Autodesk Inventor part; units mm, degrees
ref_plane "YZ Plane" through (0, 0, 0) normal (1, 0, 0) x (0, 1, 0)
ref_plane "XZ Plane" through (0, 0, 0) normal (0, 1, 0) x (-1, 0, 0)
ref_plane "XY Plane" through (0, 0, 0) normal (0, 0, 1) x (1, 0, 0)
sketch "Sketch2" plane through (0, 0, 0) normal (0, 1, 0) x (-1, 0, 0)
  line L0 (-75, -30) -> (75, -30)
  line L1 (75, -30) -> (75, 30)
  line L2 (75, 30) -> (-75, 30)
  line L3 (-75, 30) -> (-75, -30)
  line L4 (-75, -30) -> (75, 30) construction
  line L5 (75, -30) -> (-75, 30) construction
  line L6 (-84, -39) -> (84, -39)
  line L7 (84, -39) -> (84, 39)
  line L8 (84, 39) -> (-84, 39)
  line L9 (-84, 39) -> (-84, -39)
  line L10 (-84, -39) -> (84, 39) construction
  line L11 (84, -39) -> (-84, 39) construction
  point P0 (0, 0)
  dimension "d0" = 150
  dimension "d1" = 60
  dimension "d4" = 9
  dimension "d5" = 9
  dimension "d53" = 168
  dimension "d54" = 78
extrude "Extrusion1" add sketch "Sketch2" along normal blind 10
sketch "Sketch4" plane through (0, 10, 0) normal (0, 1, 0) x (1, 0, 0)
  line L0 (-84, 39) -> (-84, -39) construction
  line L1 (-84, -39) -> (84, -39) construction
  line L2 (84, -39) -> (84, 39) construction
  line L3 (84, 39) -> (-84, 39) construction
  line L4 (75, 30) -> (75, -30) construction
  line L5 (75, -30) -> (-75, -30) construction
  line L6 (-75, -30) -> (-75, 30) construction
  line L7 (-75, 30) -> (75, 30) construction
  line L8 (-75, 30) -> (75, 30)
  line L9 (75, 30) -> (75, -30)
  line L10 (75, -30) -> (-75, -30)
  line L11 (-75, -30) -> (-75, 30)
  line L12 (-75, 30) -> (75, -30) construction
  line L13 (75, 30) -> (-75, -30) construction
  line L14 (-79, 34) -> (79, 34)
  line L15 (79, 34) -> (79, -34)
  line L16 (79, -34) -> (-79, -34)
  line L17 (-79, -34) -> (-79, 34)
  line L18 (-79, 34) -> (79, -34) construction
  line L19 (79, 34) -> (-79, -34) construction
  point P0 (0, 0)
  dimension "d8" = 4
  dimension "d9" = 4
extrude "Extrusion2" cut sketch "Sketch4" against normal blind 1
sketch "Sketch7" plane through (0, 9, 0) normal (0, 1, 0) x (1, 0, 0)
  line L0 (79, -34) -> (-79, -34) construction
  line L1 (79, 34) -> (79, -34) construction
  line L2 (-79, 34) -> (79, 34) construction
  line L3 (-79, -34) -> (-79, 34) construction
  line L4 (75, 30) -> (-75, 30) construction
  line L5 (75, -30) -> (75, 30) construction
  line L6 (-75, -30) -> (75, -30) construction
  line L7 (-75, 30) -> (-75, -30) construction
  line L8 (-76, 31) -> (76, 31)
  line L9 (76, 31) -> (76, -31)
  line L10 (76, -31) -> (-76, -31)
  line L11 (-76, -31) -> (-76, 31)
  line L12 (-76, 31) -> (76, -31) construction
  line L13 (76, 31) -> (-76, -31) construction
  line L14 (-79, 34) -> (79, 34)
  line L15 (79, 34) -> (79, -34)
  line L16 (79, -34) -> (-79, -34)
  line L17 (-79, -34) -> (-79, 34)
  line L18 (-79, 34) -> (79, -34) construction
  line L19 (79, 34) -> (-79, -34) construction
  point P0 (0, 0)
  dimension "d15" = 3
  dimension "d16" = 3
extrude "Extrusion3" cut sketch "Sketch7" against normal blind 2.5
fillet "Fillet1" radius 2 8 edges at (76, 7.75, 31) (-76, 7.75, 31) (-76, 7.75, -31) (76, 7.75, -31) (75, 4.5, 30) (75, 4.5, -30) (-75, 4.5, -30) (-75, 4.5, 30)
fillet "Fillet2" radius 2 4 edges at (79, 8.25, 34) (79, 8.25, -34) (-79, 8.25, 34) (-79, 8.25, -34)
sketch "Sketch8" plane through (0, 10, 0) normal (0, 1, 0) x (1, 0, 0)
  line L0 (79, 32) -> (79, -32) construction
  arc A0 (77, -34) -> (79, -32) centre (77, -32) ccw construction
  line L1 (77, -34) -> (-77, -34) construction
  arc A1 (-79, -32) -> (-77, -34) centre (-77, -32) ccw construction
  line L2 (-79, -32) -> (-79, 32) construction
  arc A2 (-77, 34) -> (-79, 32) centre (-77, 32) ccw construction
  line L3 (-77, 34) -> (77, 34) construction
  arc A3 (79, 32) -> (77, 34) centre (77, 32) ccw construction
  line L4 (-84, 39) -> (-84, -39) construction
  line L5 (-84, -39) -> (84, -39) construction
  line L6 (84, -39) -> (84, 39) construction
  line L7 (84, 39) -> (-84, 39) construction
  line L8 (152.6, 0) -> (-152.6, 0) construction
  line L9 (0, 68.6) -> (0, -68.6) construction
  line L10 (-75, 28) -> (-75, -28) construction
  line L11 (73, 30) -> (-73, 30) construction
  line L12 (75, -28) -> (75, 28) construction
  line L13 (-73, -30) -> (73, -30) construction
  point P0 (0, 0)
  point P1 (81, -36)
  point P2 (81, 0)
  point P3 (81, 36)
  point P4 (0, 36)
  point P5 (-81, 36)
  point P6 (-81, 0)
  point P7 (-81, -36)
  point P8 (0, -36)
  dimension "d21" = 5
  dimension "d41" = 6
  dimension "d42" = 6
  dimension "d43" = 6
  dimension "d44" = 6
  dimension "d45" = 6
  dimension "d46" = 6
  dimension "d47" = 6
  dimension "d48" = 6
  dimension "d49" = 6
  dimension "d50" = 6
  dimension "d51" = 6
  dimension "d52" = 6
hole "Hole1" at (81, 10, 36) at (81, 10, 0) at (81, 10, -36) at (0, 10, -36) at (-81, 10, -36) at (-81, 10, 0) at (-81, 10, 36) at (0, 10, 36) direction (0, -1, 0) diameter 2.459 depth 8.8 tip angle 118
properties part number "P031_MonoVitreBas"
Source: CAD feature listing. Evaluate the final solid. Frame: model axes, mm. A direction names the side the tool comes from. Give positions to 0.01 mm unless a question says otherwise; leave off trailing zeros. Order: outer loops, then holes, each group sorted by start corner. A loop starts at its lowest first (then second) coordinate and runs counter-clockwise, first axis right, second up. Notation, with made-up numbers: (83.5, 54.25) -> (89.5, 54.25) arc R26 cw to (89.5, 85.25) -> close; hole circle Ø6 at (0.5, -8). An arc over 180 degrees is marked (long way). Use a Markdown table: item, result.
1) Section query B-B, the plane x = -69. Return the cut outline in (y, z).
Answer list:
| item | result |
|---|---|
| outline | (0, -39) -> (10, -39) -> (10, -34) -> (6.5, -34) -> (6.5, -31) -> (9, -31) -> (9, -30) -> (0, -30) -> close; (0, 30) -> (9, 30) -> (9, 31) -> (6.5, 31) -> (6.5, 34) -> (10, 34) -> (10, 39) -> (0, 39) -> close |
2) Reachability of faces 5 (the flat face through (79, 8, 0)), 6 (the flat face through (1, 5, -39)), 7 (the flat face through (1, 4, -30)) from +Z, -Z, +X, -X, +Y, -Y: full face, straight path, thin tool, end or side. Return the list, or none.
Answer list:
| item | result |
|---|---|
| face 5 | +Y |
| face 6 | -Z, +X, -X, +Y, -Y |
| face 7 | +Y, -Y |
3) Section query C-C, the plane z = 25. Return the cut outline in (x, y).
Answer list:
| item | result |
|---|---|
| outline | (-84, 0) -> (-75, 0) -> (-75, 9) -> (-76, 9) -> (-76, 6.5) -> (-79, 6.5) -> (-79, 10) -> (-84, 10) -> close; (75, 0) -> (84, 0) -> (84, 10) -> (79, 10) -> (79, 6.5) -> (76, 6.5) -> (76, 9) -> (75, 9) -> close |
4) Mould query, pull axis X, two halves, no side actions, for faces 1 (the flat face through (-84, 5, -1)), 2 (the flat face through (84, 5, 1)), 3 (the flat face through (-79, 8, 0)), 4 (the flat face through (-1, 5, 39)). Classes: +X half, -X half, draft (parallel to the pull), parting line (faces both ways), or undercut.
Answer list:
| item | result |
|---|---|
| face 1 | -X half |
| face 2 | +X half |
| face 3 | undercut |
| face 4 | draft |
5) Contact query for flat-ended pins moving along their axis: P1, Ø1.5, axis at x = 81, z = -36, coming from the -Y side; P2, Ø1.5, axis at x = -81, z = -36, coming from the +Y side. Output: stop coordinate, or through.
Answer list:
| item | result |
|---|---|
| P1 | y = 0 |
| P2 | y = 0.91 |
6) Ray query, line 1 along Z through (x, y) = (-19.5, 8.5); line 2 along Z through (x, y) = (81, 5.5); line 3 along X through (y, z) = (5, 36). Return the intervals inside material, ascending. Write a range as [from, to].
Answer list:
| item | result |
|---|---|
| line 1 | [-39, -34], [-31, -30], [30, 31], [34, 39] |
| line 2 | [-39, -37.23], [-34.77, -1.23], [1.23, 34.77], [37.23, 39] |
| line 3 | [-84, -82.23], [-79.77, -1.23], [1.23, 79.77], [82.23, 84] |
7) Section query A-A, the plane y = 4.5. Count the separate pieces of the cut face and the enclosed holes in it, then the cut area to 3 significant figures.
Answer list:
| item | result |
|---|---|
| separate pieces | 1 |
| enclosed holes | 9 |
| area | 4,070 mm² |
